Source: CAD feature listing. Evaluate the final solid. Frame: model axes, mm. Face numbers are marked on the shaded views. A direction names the side the tool comes from. Give positions to 0.01 mm unless a question says otherwise; leave off trailing zeros. Write each loop counter-clockwise with the first axis right and the second up, starting at its lowest first coordinate (ties: lowest second). Pieces come first, ordered by that corner, then holes. Notation, with made-up numbers: M 44.5,76 L 66.5,76 A16 ccw 66.5,98 Z; hole C 61,59.5 d8. An arc over 180 degrees is marked long. Use CSV: the item, a comma, the result in double quotes. Start each with the question number.
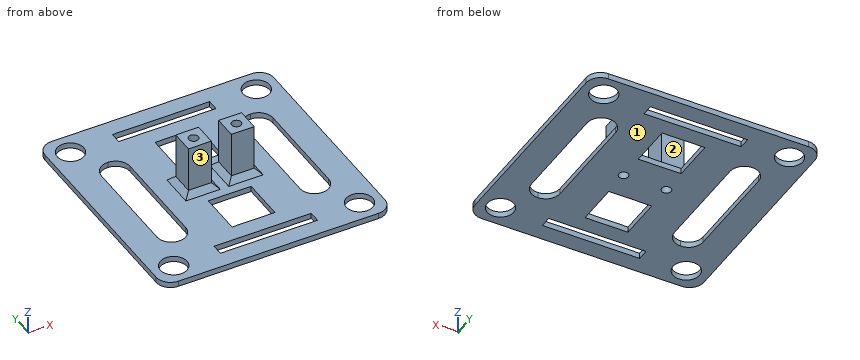
from build123d import *

# Parameters (mm, degrees)
F0_W     = 8
F0_H     = 8
F0_R     = 1.65
F1_DEPTH = 20
F0_W_2   = 80
F0_H_2   = 80
F0_R_2   = 4.65
F0_W_3   = 15
F0_H_3   = 15
F2_DEPTH = 2
F3_R     = 5
F4_SIZE  = 2
F5_SIZE  = 2
F6_SIZE  = 2
F7_SIZE  = 2
F8_W     = 34
F8_H     = 4
F9_DEPTH = 25


with BuildPart() as f1:
    # F0 (on Top) → F1 (new body)
    with BuildSketch(Plane.XY):
        with Locations((32.5, 40)):
            Rectangle(F0_W, F0_H)
        with Locations((32.5, 40)):
            Circle(F0_R, mode=Mode.SUBTRACT)
    extrude(amount=F1_DEPTH)



with BuildPart() as f1b:
    # F0 (on Top) → F1, piece 2 (new body)
    with BuildSketch(Plane.XY):
        with Locations((47.5, 40)):
            Rectangle(F0_W, F0_H)
        with Locations((47.5, 40)):
            Circle(F0_R, mode=Mode.SUBTRACT)
    extrude(amount=F1_DEPTH)


with BuildPart() as f1_1:
    add(f1.part)

    add(f1b.part)  # F2 merges F1b
    # F0 (on Top) → F2 (join)
    with BuildSketch(Plane.XY):
        with Locations((40, 40)):
            Rectangle(F0_W_2, F0_H_2)
        with Locations((7.5, 7.5)):
            Circle(F0_R_2, mode=Mode.SUBTRACT)
        with Locations((72.5, 7.5)):
            Circle(F0_R_2, mode=Mode.SUBTRACT)
        with Locations((40, 23.25)):
            Rectangle(F0_W_3, F0_H_3, mode=Mode.SUBTRACT)
        with Locations((32.5, 40)):
            Rectangle(F0_W, F0_H, mode=Mode.SUBTRACT)
        with Locations((7.5, 72.5)):
            Circle(F0_R_2, mode=Mode.SUBTRACT)
        with Locations((47.5, 40)):
            Rectangle(F0_W, F0_H, mode=Mode.SUBTRACT)
        with Locations((40, 56.75)):
            Rectangle(F0_W_3, F0_H_3, mode=Mode.SUBTRACT)
        with Locations((72.5, 72.5)):
            Circle(F0_R_2, mode=Mode.SUBTRACT)
    extrude(amount=F2_DEPTH)

    # F3
    f3_edges = [f1_1.edges().sort_by_distance(p)[0] for p in [
        (0, 80, 1),
        (80, 80, 1),
        (80, 0, 1),
        (0, 0, 1),
    ]]
    fillet(f3_edges, radius=F3_R)

    # F4
    f4_edges = [f1_1.edges().sort_by_distance(p)[0] for p in [
        (32.5, 44, 2),
        (47.5, 44, 2),
    ]]
    chamfer(f4_edges, length=F4_SIZE)

    # F5
    f5_edges = [f1_1.edges().sort_by_distance(p)[0] for p in [
        (32.5, 36, 2),
        (47.5, 36, 2),
    ]]
    chamfer(f5_edges, length=F5_SIZE)

    # F6
    f6_edges = [f1_1.edges().sort_by_distance(p)[0] for p in [
        (28.5, 40, 2),
        (36.5, 40, 2),
    ]]
    chamfer(f6_edges, length=F6_SIZE)

    # F7
    f7_edges = [f1_1.edges().sort_by_distance(p)[0] for p in [
        (51.5, 40, 2),
        (43.5, 40, 2),
    ]]
    chamfer(f7_edges, length=F7_SIZE)

    # F8 (on face) → F9 (cut)
    with BuildSketch(Plane.XY.offset(2)):
        with BuildLine():
            Line((20, 22.5), (20, 57.5))
            ThreePointArc((20, 57.5), (18.5355339059, 61.0355339059), (15, 62.5))
            ThreePointArc((15, 62.5), (11.4644660941, 61.0355339059), (10, 57.5))
            Line((10, 57.5), (10, 22.5))
            ThreePointArc((10, 22.5), (11.4644660941, 18.9644660941), (15, 17.5))
            ThreePointArc((15, 17.5), (18.5355339059, 18.9644660941), (20, 22.5))
        make_face()
        with BuildLine():
            ThreePointArc((65, 62.5), (61.4644660941, 61.0355339059), (60, 57.5))
            Line((60, 57.5), (60, 22.5))
            ThreePointArc((60, 22.5), (61.4644660941, 18.9644660941), (65, 17.5))
            ThreePointArc((65, 17.5), (68.5355339059, 18.9644660941), (70, 22.5))
            Line((70, 22.5), (70, 57.5))
            ThreePointArc((70, 57.5), (68.5355339059, 61.0355339059), (65, 62.5))
        make_face()
        with Locations((40, 72)):
            Rectangle(F8_W, F8_H)
        with Locations((40, 8)):
            Rectangle(F8_W, F8_H)
    extrude(amount=-F9_DEPTH, mode=Mode.SUBTRACT)


solid = f1_1.part
1. Section D-D on y = 40. Give the number of separate pieces and of enclosed holes in the cut face, then the cut area to 3 significant figures.
2. Line query: probe 1 along Y at (x, z) = (7.5, 0.7); probe 2 along Y at (x, z) = (35, 1.5); probe 3 along Y at (x, z) = (47.5, 10.75). Output: solid intervals per line, ascending.
3. Access query for the marked faces 1, 2 and 3. Directions: +Z, -Z, +X, -X, +Y, -Y. A direction counts if a zero-diameter tool reaches every point of the face in a straight line with its end or side. Return the directions, or none.
4. Section C-C on x = 39.5. Return loops of the section in (y, z).
5. Section A-A on z = 9. Return loops of the section in (x, y).
6. First-contact query: pin 1 (2.5 mm diameter, centred on x = 32.5, y = 40, fed in from +Z); pin 2 (2.5 mm diameter, centred on x = 33, z = 15.5, fed in from -Y); pin 3 (6.5 mm diameter, centred on y = 40, z = 9, fed in from +X); pin 4 (12 mm diameter, centred on x = 7.5, y = 7.5, fed in from -Z). Flat tips, straight axial feed; report the tip coordinate or a pass-through.
7. Section B-B on y = 7.5. Return loops of the section in (x, z), then the cut area to 3 significant figures.
Resolved:
1,separate pieces,"5"
1,enclosed holes,"0"
1,area,"284 mm2"
2,probe 1,"y = 0 to 2.85, 12.15 to 67.85, 77.15 to 80"
2,probe 2,"y = 0 to 6, 10 to 15.75, 30.75 to 49.25, 64.25 to 70, 74 to 80"
2,probe 3,"y = 36 to 38.35, 41.65 to 44"
3,face 1,"-Z, +X, -X, +Y, -Y"
3,face 2,"+Z, +X, -X, +Y"
3,face 3,"+Z, +X, -X, -Y"
4,outline,"M 0,0 L 6,0 L 6,2 L 0,2 Z; M 10,0 L 15.75,0 L 15.75,2 L 10,2 Z; M 30.75,0 L 49.25,0 L 49.25,2 L 30.75,2 Z; M 64.25,0 L 70,0 L 70,2 L 64.25,2 Z; M 74,0 L 80,0 L 80,2 L 74,2 Z"
5,outline,"M 28.5,36 L 36.5,36 L 36.5,44 L 28.5,44 Z; M 43.5,36 L 51.5,36 L 51.5,44 L 43.5,44 Z; hole C 32.5,40 d3.3; hole C 47.5,40 d3.3"
6,pin 1,"passes through"
6,pin 2,"stops at y = 36"
6,pin 3,"stops at x = 51.5"
6,pin 4,"stops at z = 0"
7,outline,"M 0,0 L 2.85,0 L 2.85,2 L 0,2 Z; M 12.15,0 L 23,0 L 23,2 L 12.15,2 Z; M 57,0 L 67.85,0 L 67.85,2 L 57,2 Z; M 77.15,0 L 80,0 L 80,2 L 77.15,2 Z"
7,area,"54.8 mm2"
